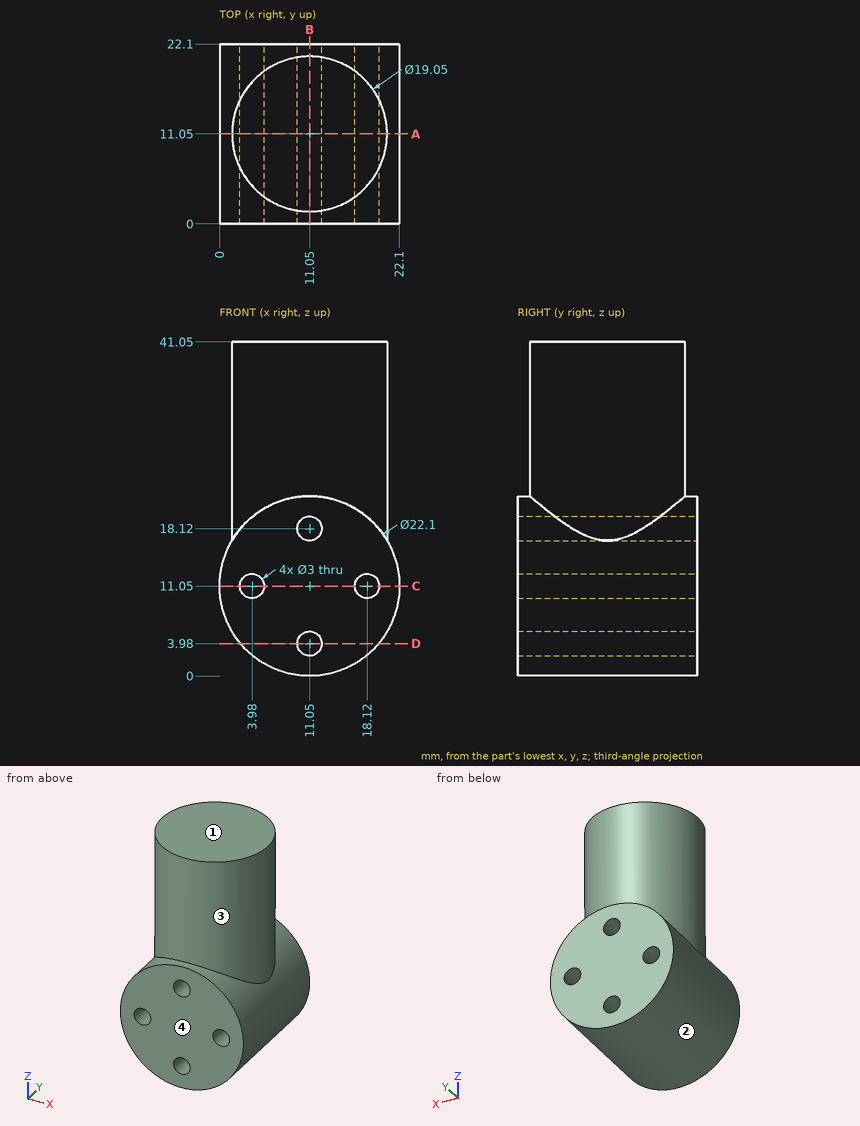
Source: three-view drawing plus pictorial views. Frame: mm from the lowest corner of the part. A direction names the side the tool comes from. Give positions to 0.01 mm unless a question says otherwise; leave off trailing zeros. Order: outer loops, then holes, each group sorted by start corner. A loop starts at its lowest first (then second) coordinate and runs counter-clockwise, first axis right, second up. Notation, with made-up numbers: M 57,-34.5 L 63,-34.5 A21 cw 63,-9.5 Z; hole C 28,30.5 d3. An arc over 180 degrees is marked long. Return JSON: item names as keys, results as strings.
Item 1: First-contact query: P1, Ø3, axis at y = 17.5, z = 19, coming from the -X side; P2, Ø1.5, axis at y = 11, z = 33, coming from the +X side (3 decimals); P3, Ø10, axis at y = 12.5, z = 23, coming from the -X side (3 decimals). Flat tips, straight axial feed; report the tip coordinate or a pass-through.
Solutions:
{"P1": "x = 2.08", "P2": "x = 20.575", "P3": "x = 1.525"}
Item 2: Cut plane C-C (z = 11.05). Return loops of the section in (x, y), then the cut area to 3 significant figures.
Solutions:
{"outline": "M 0,0 L 2.48,0 L 2.48,22.1 L 0,22.1 Z; M 5.48,0 L 16.62,0 L 16.62,22.1 L 5.48,22.1 Z; M 19.62,0 L 22.1,0 L 22.1,22.1 L 19.62,22.1 Z", "area": "356 mm^2"}
Item 3: Cut plane D-D (z = 3.98). Return loops of the section in (x, y).
Solutions:
{"outline": "M 2.56,0 L 9.55,0 L 9.55,22.1 L 2.56,22.1 Z; M 12.55,0 L 19.54,0 L 19.54,22.1 L 12.55,22.1 Z"}
Item 4: Cut plane B-B (x = 11.05). Return loops of the section in (y, z) (3 decimals).
Solutions:
{"outline": "M 0,0 L 22.1,0 L 22.1,2.48 L 0,2.48 Z; M 0,5.48 L 22.1,5.48 L 22.1,16.62 L 0,16.62 Z; M 0,19.62 L 22.1,19.62 L 22.1,22.1 L 20.575,22.1 L 20.575,41.05 L 1.525,41.05 L 1.525,22.1 L 0,22.1 Z"}
Item 5: Ray query, probe 1 along Z at (x, y) = (10.5, 17.75); probe 2 along X at (y, z) = (16.75, 3); probe 3 along Z at (x, y) = (18.12, 11.75). Return the intervals inside material, ascending.
Solutions:
{"probe 1": "0.01 to 2.58, 5.38 to 16.72, 19.52 to 41.05", "probe 2": "3.48 to 9.91, 12.19 to 18.62", "probe 3": "2.56 to 9.55, 12.55 to 41.05"}
Item 6: Pull-direction query (X, two-part tool) for the marked faces 1 and 2; classes: +X half, -X half, draft (parallel to the pull), parting line (faces both ways), or undercut.
Solutions:
{"face 1": "draft", "face 2": "parting line"}
Item 7: Cut plane A-A (y = 11.05). State how many separate pieces and enclosed holes the cut face has, then the cut area to 3 significant figures.
Solutions:
{"separate pieces": "1", "enclosed holes": "4", "area": "747 mm^2"}
Item 8: Access query for the marked faces 3 and 4. Directions: +Z, -Z, +X, -X, +Y, -Y. A direction counts if a zero-diameter tool reaches every point of the face in a straight line with its end or side. Return the directions, or none.
Solutions:
{"face 3": "+Z", "face 4": "+Z, -Z, +X, -X, -Y"}
